from build123d import *

# Parameters (mm, degrees)
ESCALA1_SCALE               = 0.2
PADR_OCIRCULAR1_COUNT       = 4
FURO_COM_FOLGA_DE_M61_D     = 6.6
FURO_COM_FOLGA_DE_M61_DEPTH = 19.342621622
FURO_COM_FOLGA_DE_M61_TIP   = 1.982840043


with BuildPart() as part:
    # Esboço1 → Revolução1 (revolve)
    with BuildSketch(Plane.XY, mode=Mode.PRIVATE) as revolu_o1_sk:
        with BuildLine():
            Line((3250.53685571, 0), (3250.53685571, 383.5))
            Line((3250.53685571, 383.5), (2198.53685571, 873))
            Line((2198.53685571, 873), (746.53685571, 1260))
            ThreePointArc((746.53685571, 1260), (705.413382944, 1272.149939556), (665, 1286.485891657))
            ThreePointArc((665, 1286.485891657), (0, 1410.13859172), (-665, 1286.485891657))
            ThreePointArc((-665, 1286.485891657), (-700.329808436, 1276.488395428), (-736.891891892, 1273.118032191))
            Line((-736.891891892, 1273.118032191), (-736.891891892, 1244.476357536))
            Line((-736.891891892, 1244.476357536), (41.718108108, 1244.476357536))
            Line((41.718108108, 1244.476357536), (41.718108108, 1164.476357536))
            Line((41.718108108, 1164.476357536), (71.718108108, 1164.476357536))
            Line((71.718108108, 1164.476357536), (71.718108108, 1244.476357536))
            Line((71.718108108, 1244.476357536), (746.53685571, 1244.476357536))
            Line((746.53685571, 1244.476357536), (1303.338284236, 1096.072671007))
            Line((1303.338284236, 1096.072671007), (2193.402058482, 858.844929525))
            Line((2193.402058482, 858.844929525), (3235.53685571, 373.935249636))
            Line((3235.53685571, 373.935249636), (3235.53685571, 0))
            Line((3235.53685571, 0), (3250.53685571, 0))
        make_face()
    revolve(revolu_o1_sk.sketch.rotate(Axis((-169.437422306, 0, 0), (1, 0, 0)), 90), axis=Axis((-169.437422306, 0, 0), (1, 0, 0)))


with BuildPart() as part_1:
    # Escala1: scaled about (0, 0, 0)
    add(part.part.scale(ESCALA1_SCALE))

    # Esboço2 → Corte-Revolução9 (revolve, cut)
    with BuildSketch(Plane.XY, mode=Mode.PRIVATE) as corte_revolu_o9_sk:
        Polygon((15, 268.895271507), (15, 263.895271507), (0, 263.895271507), (0, 311.146389703), (175.532983409, 311.146389703), (175.532983409, 253.895271507), (50, 253.895271507), (50, 268.895271507), align=None)
    corte_revolu_o9 = revolve(corte_revolu_o9_sk.sketch.rotate(Axis((0, -141.14012245, 0), (0, 1, 0)), 90), axis=Axis((0, -141.14012245, 0), (0, 1, 0)), mode=Mode.SUBTRACT)

    # PadrãoCircular1: Corte-Revolução9 ×4 about axis
    padr_ocircular1_axis = Axis((0, 0, 0), (1, 0, 0))
    for i in range(1, PADR_OCIRCULAR1_COUNT):
        add(corte_revolu_o9.rotate(padr_ocircular1_axis, i * 360 / PADR_OCIRCULAR1_COUNT), mode=Mode.SUBTRACT)

    # Furo com folga de M61
    with Locations(Plane(origin=(14.343621622, 0, 0), x_dir=(0, 0, -1), z_dir=(1, 0, 0))):
        with Locations((0, 240.895271507), (240.895271507, 0), (0, -240.895271507), (-240.895271507, 0), (0, 0)):
            Hole(FURO_COM_FOLGA_DE_M61_D / 2, depth=FURO_COM_FOLGA_DE_M61_DEPTH)
            with Locations((0, 0, -(FURO_COM_FOLGA_DE_M61_DEPTH + FURO_COM_FOLGA_DE_M61_TIP / 2))):  # 118° drill point
                Cone(0, FURO_COM_FOLGA_DE_M61_D / 2, FURO_COM_FOLGA_DE_M61_TIP, mode=Mode.SUBTRACT)


solid = part_1.part
Source: CAD feature listing. Evaluate the final solid. Frame: model axes, mm. A direction names the side the tool comes from. Coordinates: 2 decimals unless noted, no trailing zeros. Order: outer loops, then holes, each group sorted by start corner. A loop starts at its lowest first (then second) coordinate and runs counter-clockwise, first axis right, second up. Notation, with made-up numbers: M 66.5,-4.5 L 109.5,-4.5 A29 ccw 109.5,23.5 Z; hole C -20.5,-31.5 d7. An arc over 180 degrees is marked long. Write each question's results on one line, items separated by ' | '. Start each with the question number.
Item 1: Draft query along Y for faces 1 (the face through (0, 0, -263.895)), 2 (the face through (0, 263.895, 0)), 3 (the face through (-4, -253.895, 53)), 4 (the face through (11.39, -69.96, 222.14)). Return one class per face: pulls with the +Y half, pulls with the -Y half, needs draft (parallel to the pull), parting line crosses it, or undercut.
Item 2: First-contact query: pin 1 Ø5 at (x, z) = (-29, 131) entering from -Y; pin 2 Ø4 at (y, z) = (24, -26.5) entering from -X; pin 3 Ø1.5 at (x, y) = (-56, 70.5) entering from +Z. Flat tips, straight axial feed; report the tip coordinate or a pass-through.
Item 3: Set-up query: faces 5 (the face through (-4, -53, -253.895)), 6 (the face through (8.344, 165, 165)), 7 (the face through (0, -263.895, 0)), 8 (the face through (-0.66, -14.985, 266.36)), 9 (the face through (82.77, -246.777, -32.401)). Return all of +Z, -Z, +X, -X, +Y, -Y with unobstructed straight access to the full face (end or side cutting, diameter ignored); none if empty.
Item 4: Cut plane B-B (x = 549.5). Return loops of the section in (y, z).
Item 5: Cut plane A-A (x = 297). Return loops of the section in (y, z).
Item 6: Line query: probe 1 along Y at (x, z) = (10.5, 0); probe 2 along X at (y, z) = (0, 265.9); probe 3 along Z at (x, y) = (69.5, -202). Output: solid intervals per line, ascending.
Checked values:
1) face 1: undercut | face 2: pulls with the +Y half | face 3: pulls with the -Y half | face 4: undercut
2) pin 1: stops at y = -249.79 | pin 2: stops at x = 647.11 | pin 3: stops at z = 253.9
3) face 5: -Z | face 6: -X | face 7: -Y | face 8: +Z | face 9: none
4) outline: C 0,0 d247.03; hole C 0,0 d240.41
5) outline: C 0,0 d425.27; hole C 0,0 d419.06
6) probe 1: y = -263.9 to -244.2, -237.6 to -232.9, 232.9 to 237.6, 244.2 to 263.9 | probe 2: x = -50 to -15, 15 to 50 | probe 3: z = -187.25 to -145.41, 145.41 to 187.25
